from build123d import *


with BuildPart() as part:
    # Sweep1: sweep along a path in Sketch2
    with BuildLine(Plane(origin=(0, 0, 0), x_dir=(1, 0, 0), z_dir=(0, 1, 0))) as sweep1_path:
        Line((-409.575, 0), (-409.575, -152.4))
        Line((-409.575, -152.4), (409.575, -152.4))
        Line((409.575, -152.4), (409.575, 0))
    # Sketch1 → Sweep1 (sweep)
    with BuildSketch(Plane.XY):
        with BuildLine():
            Line((-428.625, 127), (-460.375, 127))
            ThreePointArc((-460.375, 127), (-482.825640303, 117.700640303), (-492.125, 95.25))
            Line((-492.125, 95.25), (-492.125, 31.75))
            ThreePointArc((-492.125, 31.75), (-482.825640303, 9.299359697), (-460.375, 0))
            Line((-460.375, 0), (-428.625, 0))
            Line((-428.625, 0), (-409.575, 0))
            Line((-409.575, 0), (-409.575, 127))
            Line((-409.575, 127), (-428.625, 127))
        make_face()
    sweep(path=sweep1_path.line, transition=Transition.RIGHT)


solid = part.part
Geometry check sheet. Reference: the model listing, model coordinates, mm. A direction names the side the tool comes from. Round coordinates to 2 decimals unless told otherwise and drop trailing zeros. Loops run counter-clockwise (first coordinate to the right, second up) from the corner with the lowest first, then second, coordinate; pieces in that order, holes last.
Item 1: Cross-section at A-A on z = 110. Record the boundary of the cut face in (x, y) (3 decimals), then the cut area to 3 significant figures.
Item 2: Cross-section at D-D on y = 109.5. Record the boundary of the cut face in (x, z) (3 decimals).
Item 3: Mould release check, pull along X, two halves, no side actions. Record for faces 1 (the flat face through (409.575, 63, 75)), 2 (the cylindrical face through (482.577, 117.946, 115.83)), 3 (the cylindrical face through (6.89, 9.55, 225.9)): pulls with the +X half, pulls with the -X half, needs draft (parallel to the pull), parting line crosses it, or undercut.
Item 4: Cross-section at C-C on x = -379.5. Record the boundary of the cut face in (y, z), then the cut area to 3 significant figures.
Item 5: Cross-section at B-B on y = 51. Record the boundary of the cut face in (x, z) (3 decimals).
Item 6: Gauge pin test, flat end, axial feed: pin 1 (8 mm diameter, centred on x = 197, y = 87, fed in from -Z). Record the tip position at first contact, or that the pin passes through.
Item 7: Access from +Z, -Z, +X, -X, +Y, -Y to the whole of each face (thin tool, end or side, straight path). Record for faces 4 (the flat face through (6, 63, 152.4)), 5 (the flat face through (492.125, 64, 116)).
Item 8: Thickness scan on line 1 (Z direction, x = -13.5, y = 47); line 2 (X direction, y = 69.5, z = 106) (3 decimals); line 3 (X direction, y = 17.5, z = 120.5) (3 decimals). Record the ranges inside material, lowest first.
Answer sheet:
1. outline: (-492.125, 31.75) arc R31.75 ccw to (-460.375, 0) - (-409.575, 0) - (-409.575, 127) - (-460.375, 127) arc R31.75 ccw to (-492.125, 95.25) - close; (409.575, 0) - (460.375, 0) arc R31.75 ccw to (492.125, 31.75) - (492.125, 95.25) arc R31.75 ccw to (460.375, 127) - (409.575, 127) - close
1. area: 20,100 mm2
2. outline: (-488.748, 0) - (-409.575, 0) - (-409.575, 152.4) - (409.575, 152.4) - (409.575, 0) - (488.748, 0) - (488.748, 231.573) - (-488.748, 231.573) - close
3. face 1: undercut
3. face 2: pulls with the +X half
3. face 3: needs draft
4. outline: (0, 152.4) - (127, 152.4) - (127, 203.2) arc R31.75 ccw to (95.25, 234.95) - (31.75, 234.95) arc R31.75 ccw to (0, 203.2) - close
4. area: 10,100 mm2
5. outline: (-492.125, 0) - (-409.575, 0) - (-409.575, 152.4) - (409.575, 152.4) - (409.575, 0) - (492.125, 0) - (492.125, 234.95) - (-492.125, 234.95) - close
6. pin 1: stops at z = 152.4
7. face 4: -Z, +Y, -Y
7. face 5: +Z, -Z, +X, +Y, -Y
8. line 1: z = 152.4 to 234.95
8. line 2: x = -492.125 to -409.575, 409.575 to 492.125
8. line 3: x = -488.748 to -409.575, 409.575 to 488.748
